```python
from build123d import *

# Parameters (mm, degrees)
PAD_DEPTH        = 20
HOLE_D           = 3.5
HOLE_CSINK_D     = 8
HOLE_CSINK_ANGLE = 90


with BuildPart() as part:
    # Sketch → Pad (new body, symmetric)
    with BuildSketch(Plane.YZ):
        with BuildLine():
            ThreePointArc((39.39231, 18.945927), (37.587705, 25.680806), (34.641016, 32))
            Line((34.641016, 32), (47.631397, 39.5))
            Line((47.631397, 59.5), (47.631397, 39.5))
            Line((50.560329, 59.5), (47.631397, 59.5))
            Line((50.560329, 59.5), (52.631397, 57.428932))
            Line((52.631397, 21.280335), (52.631397, 57.428932))
            Line((39.39231, 18.945927), (52.631397, 21.280335))
        make_face()
    extrude(amount=PAD_DEPTH, both=True)

    # Hole (through all)
    with Locations(Plane.ZX.offset(52.631397)):
        with Locations((49.5, 0)):
            CounterSinkHole(HOLE_D / 2, HOLE_CSINK_D / 2, counter_sink_angle=HOLE_CSINK_ANGLE)


solid = part.part
```
Check sheet for the modelled part. Datum: model origin and axes. Units: mm. A direction names the side the tool comes from. Give positions to 0.01 mm unless a question says otherwise; leave off trailing zeros. Write each loop counter-clockwise with the first axis right and the second up, starting at its lowest first coordinate (ties: lowest second). Pieces come first, ordered by that corner, then holes. Notation, with made-up numbers: (6, 59.5) - (10, 59.5) arc R20 ccw to (10, 69.5) - close; hole circle Ø4 at (65, 88). An arc over 180 degrees is marked (long way). Answer as a JSON object with one key per item and string values. Group by question number.
1) Sectioned sample at C-C (y = 48.75). Record the cut outline in (x, z).
2) Sectioned sample at A-A (z = 49.5). Record the cut outline in (x, y), then the cut area to 3 significant figures.
3) Release check for a two-part mould opening along Z. For faces 3 (the face through (0.56, 50.49, 47.73)), 4 (the face through (0.28, 41.05, 35.7)), 5 (the face through (0, 52.631, 39)) record: pulls with the +Z half, pulls with the -Z half, needs draft (parallel to the pull), parting line crosses it, or undercut.
4) Sectioned sample at D-D (z = 24). Record the cut outline in (x, y).
5) Sectioned sample at B-B (x = 11). Record the cut outline in (y, z).
6) Access from +Z, -Z, +X, -X, +Y, -Y to the whole of each face (thin tool, end or side, straight path). Record for faces 1 (the face through (-20, 46, 35)), 2 (the face through (0, 47.631, 47)).
7) Depth check by flat-ended pin: P1, Ø6, axis at x = -10, y = 37.5, coming from the -Z side; P2, Ø8, axis at x = -16, z = 26.5, coming from the -Y side; P3, Ø10, axis at x = 2, z = 52, coming from the -Y side; P4, Ø2, axis at x = 0, z = 49.5, coming from the -Y side. Enter the tip coordinate at first touch or a pass-through.
8) Thickness scan on probe 1 along X at (y, z) = (49.8, 49.5); probe 2 along Z at (x, y) = (0, 49.5); probe 3 along Z at (x, y) = (0, 48.5). Record the ranges inside material, lowest first. Write a range as from..to.
Geometry results:
{
 "1": {"outline": "(-20, 20.6) - (20, 20.6) - (20, 59.5) - (-20, 59.5) - close; hole circle Ø3.5 at (0, 49.5)"},
 "2": {"outline": "(-20, 47.63) - (-1.75, 47.63) - (-1.75, 50.38) - (-4, 52.63) - (-20, 52.63) - close; (1.75, 47.63) - (20, 47.63) - (20, 52.63) - (4, 52.63) - (1.75, 50.38) - close", "area": "177 mm^2"},
 "3": {"face 3": "undercut", "face 4": "pulls with the +Z half", "face 5": "needs draft"},
 "4": {"outline": "(-20, 38.16) - (20, 38.16) - (20, 52.63) - (-20, 52.63) - close"},
 "5": {"outline": "(34.64, 32) arc R40 cw to (39.39, 18.95) - (52.63, 21.28) - (52.63, 57.43) - (50.56, 59.5) - (47.63, 59.5) - (47.63, 39.5) - close"},
 "6": {"face 1": "+Z, -Z, -X, +Y, -Y", "face 2": "+Z, +X, -X, -Y"},
 "7": {"P1": "stops at z = 18.95", "P2": "stops at y = 35.46", "P3": "stops at y = 47.63", "P4": "passes through"},
 "8": {"probe 1": "x = -20..-1.75, 1.75..20", "probe 2": "z = 20.73..47.75, 51.25..59.5", "probe 3": "z = 20.55..47.75, 51.25..59.5"}
}
